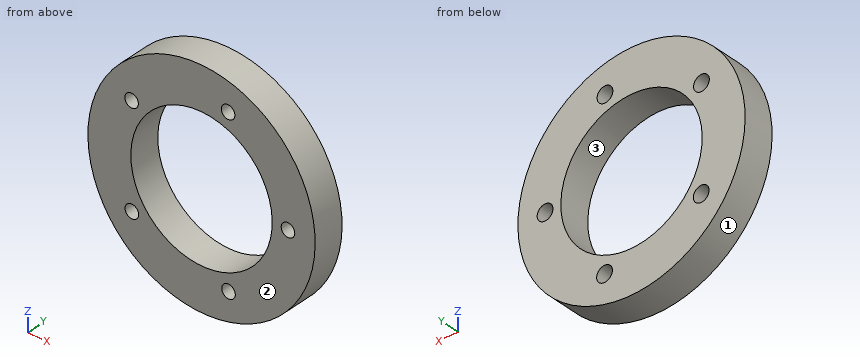
```python
from build123d import *

# Parameters (mm, degrees)
SKETCH1_R                    = 16.2
SKETCH1_R_2                  = 11.2
BOSS_EXTRUDE2_DEPTH          = 5
SKETCH2_R                    = 1.25
CUT_EXTRUDE1_DEPTH           = 5
CUT_EXTRUDE1_DRAFT           = -2
CUT_EXTRUDE1_PROFILE_2_DEPTH = 5
CUT_EXTRUDE1_PROFILE_2_DRAFT = -2
CUT_EXTRUDE1_PROFILE_3_DEPTH = 5
CUT_EXTRUDE1_PROFILE_3_DRAFT = -2
CUT_EXTRUDE1_PROFILE_4_DEPTH = 5
CUT_EXTRUDE1_PROFILE_4_DRAFT = -2
CUT_EXTRUDE1_PROFILE_5_DEPTH = 5
CUT_EXTRUDE1_PROFILE_5_DRAFT = -2
SKETCH3_R                    = 18
SKETCH3_R_2                  = 16
BOSS_EXTRUDE4_DEPTH          = 5


with BuildPart() as part:
    # Sketch1 → Boss-Extrude2 (new body)
    with BuildSketch(Plane(origin=(0, 0, 0), x_dir=(1, 0, 0), z_dir=(0, 1, 0))):
        with Locations(Location((0, 0, 0), (0, 0, 270))):
            Circle(SKETCH1_R)
        with Locations(Location((0, 0, 0), (0, 0, 270))):
            Circle(SKETCH1_R_2, mode=Mode.SUBTRACT)
    extrude(amount=BOSS_EXTRUDE2_DEPTH)


with BuildPart() as cut_extrude1_tool:
    # Sketch2 → Cut-Extrude1 (with draft: the straight prism first)
    with BuildSketch(Plane(origin=(0, 5, 0), x_dir=(1, 0, 0), z_dir=(0, 1, 0))):
        with Locations((-11.039322132, 8.113160104)):
            Circle(SKETCH2_R)
    extrude(amount=-CUT_EXTRUDE1_DEPTH)
    # Cut-Extrude1: the draft: its side faces are tilted about the plane it starts from
    cut_extrude1_sides = [cut_extrude1_tool.faces().sort_by_distance(p)[0] for p in [
        (-12.289322132, 2.5, -8.113160104),
    ]]
    draft(cut_extrude1_sides, Plane(origin=(0, 5, 0), x_dir=(1, 0, 0), z_dir=(0, 1, 0)), CUT_EXTRUDE1_DRAFT)


with BuildPart() as part_1:
    add(part.part)

    # Cut-Extrude1: cut by cut_extrude1_tool
    add(cut_extrude1_tool.part, mode=Mode.SUBTRACT)


with BuildPart() as cut_extrude1_profile_2_tool:
    # Sketch2 → Cut-Extrude1 profile 2 (with draft: the straight prism first)
    with BuildSketch(Plane(origin=(0, 5, 0), x_dir=(1, 0, 0), z_dir=(0, 1, 0))):
        with Locations((-11.083327892, -7.977724299)):
            Circle(SKETCH2_R)
    extrude(amount=-CUT_EXTRUDE1_PROFILE_2_DEPTH)
    # Cut-Extrude1 profile 2: the draft: its side faces are tilted about the plane it starts from
    cut_extrude1_profile_2_sides = [cut_extrude1_profile_2_tool.faces().sort_by_distance(p)[0] for p in [
        (-12.333327892, 2.5, 7.977724299),
    ]]
    draft(cut_extrude1_profile_2_sides, Plane(origin=(0, 5, 0), x_dir=(1, 0, 0), z_dir=(0, 1, 0)), CUT_EXTRUDE1_PROFILE_2_DRAFT)


with BuildPart() as part_2:
    add(part_1.part)

    # Cut-Extrude1 profile 2: cut by cut_extrude1_profile_2_tool
    add(cut_extrude1_profile_2_tool.part, mode=Mode.SUBTRACT)


with BuildPart() as cut_extrude1_profile_3_tool:
    # Sketch2 → Cut-Extrude1 profile 3 (with draft: the straight prism first)
    with BuildSketch(Plane(origin=(0, 5, 0), x_dir=(1, 0, 0), z_dir=(0, 1, 0))):
        with Locations((4.206414044, -12.991932999)):
            Circle(SKETCH2_R)
    extrude(amount=-CUT_EXTRUDE1_PROFILE_3_DEPTH)
    # Cut-Extrude1 profile 3: the draft: its side faces are tilted about the plane it starts from
    cut_extrude1_profile_3_sides = [cut_extrude1_profile_3_tool.faces().sort_by_distance(p)[0] for p in [
        (2.956414044, 2.5, 12.991932999),
    ]]
    draft(cut_extrude1_profile_3_sides, Plane(origin=(0, 5, 0), x_dir=(1, 0, 0), z_dir=(0, 1, 0)), CUT_EXTRUDE1_PROFILE_3_DRAFT)


with BuildPart() as part_3:
    add(part_2.part)

    # Cut-Extrude1 profile 3: cut by cut_extrude1_profile_3_tool
    add(cut_extrude1_profile_3_tool.part, mode=Mode.SUBTRACT)


with BuildPart() as cut_extrude1_profile_4_tool:
    # Sketch2 → Cut-Extrude1 profile 4 (with draft: the straight prism first)
    with BuildSketch(Plane(origin=(0, 5, 0), x_dir=(1, 0, 0), z_dir=(0, 1, 0))):
        with Locations((13.7, 0)):
            Circle(SKETCH2_R)
    extrude(amount=-CUT_EXTRUDE1_PROFILE_4_DEPTH)
    # Cut-Extrude1 profile 4: the draft: its side faces are tilted about the plane it starts from
    cut_extrude1_profile_4_sides = [cut_extrude1_profile_4_tool.faces().sort_by_distance(p)[0] for p in [
        (12.45, 2.5, 0),
    ]]
    draft(cut_extrude1_profile_4_sides, Plane(origin=(0, 5, 0), x_dir=(1, 0, 0), z_dir=(0, 1, 0)), CUT_EXTRUDE1_PROFILE_4_DRAFT)


with BuildPart() as part_4:
    add(part_3.part)

    # Cut-Extrude1 profile 4: cut by cut_extrude1_profile_4_tool
    add(cut_extrude1_profile_4_tool.part, mode=Mode.SUBTRACT)


with BuildPart() as cut_extrude1_profile_5_tool:
    # Sketch2 → Cut-Extrude1 profile 5 (with draft: the straight prism first)
    with BuildSketch(Plane(origin=(0, 5, 0), x_dir=(1, 0, 0), z_dir=(0, 1, 0))):
        with Locations((4.27761686, 13.043664873)):
            Circle(SKETCH2_R)
    extrude(amount=-CUT_EXTRUDE1_PROFILE_5_DEPTH)
    # Cut-Extrude1 profile 5: the draft: its side faces are tilted about the plane it starts from
    cut_extrude1_profile_5_sides = [cut_extrude1_profile_5_tool.faces().sort_by_distance(p)[0] for p in [
        (3.02761686, 2.5, -13.043664873),
    ]]
    draft(cut_extrude1_profile_5_sides, Plane(origin=(0, 5, 0), x_dir=(1, 0, 0), z_dir=(0, 1, 0)), CUT_EXTRUDE1_PROFILE_5_DRAFT)


with BuildPart() as part_5:
    add(part_4.part)

    # Cut-Extrude1 profile 5: cut by cut_extrude1_profile_5_tool
    add(cut_extrude1_profile_5_tool.part, mode=Mode.SUBTRACT)

    # Sketch3 → Boss-Extrude4 (add)
    with BuildSketch(Plane(origin=(0, 5, 0), x_dir=(1, 0, 0), z_dir=(0, 1, 0))):
        with Locations(Location((0, 0, 0), (0, 0, 270))):
            Circle(SKETCH3_R)
        Circle(SKETCH3_R_2, mode=Mode.SUBTRACT)
    extrude(amount=-BOSS_EXTRUDE4_DEPTH)


solid = part_5.part
```
The listing builds one solid part. Answer for the finished solid, in the listing's coordinates (mm). Face numbers are marked on the shaded views. Give positions to 0.01 mm unless a question says otherwise; leave off trailing zeros. Order: outer loops, then holes, each group sorted by start corner. A loop starts at its lowest first (then second) coordinate and runs counter-clockwise, first axis right, second up. Notation, with made-up numbers: M 62.25,70.25 L 94.25,70.25 A7 cw 94.25,74.25 Z; hole C 86.25,38.25 d9. An arc over 180 degrees is marked long. Put each result on its own line as item: value. Start each with the question number.
Item 1: Flat-ended cylindrical pins translate along their axes: P1, Ø2, axis at y = 2, z = -10.5, coming from the -X side; P2, Ø2, axis at x = -1.5, y = 4.5, coming from the -Z side; P3, Ø1.5, axis at x = 14, y = 4, coming from the +Z side. Find the tip coordinate at first contact, or state that the pin passes through.
Item 2: The part is cut by section A-A, the plane x = 0. Determine the outline of the cut face in (y, z), and give its area (3 significant figures).
Item 3: The part is cut by section D-D, the plane z = -4. Determine the outline of the cut face in (x, y), and give its area (3 significant figures).
Item 4: The part is cut by section C-C, the plane y = 3.25. Determine the outline of the cut face in (x, z), and give its area (3 significant figures).
Item 5: The part is cut by section B-B, the plane z = 0. Determine the outline of the cut face in (x, y).
Item 6: Find the intervals of material crossed by line 1 along X through (y, z) = (3.05, 0); line 2 along X through (y, z) = (1.15, 0); line 3 along X through (y, z) = (2.25, -6), in increasing order.
Item 7: For a pull along X with two mould halves and no side action, classify the marked faces 1, 2 and 3 as +X half, -X half, draft (parallel to the pull), parting line (faces both ways), or undercut.
Answer key:
1. P1: stops at x = -15.29
1. P2: stops at z = -17.99
1. P3: stops at z = 12.18
2. outline: M 0,-18 L 5,-18 L 5,-11.2 L 0,-11.2 Z; M 0,11.2 L 5,11.2 L 5,18 L 0,18 Z
2. area: 68.0 mm²
3. outline: M -17.55,0 L -10.46,0 L -10.46,5 L -17.55,5 Z; M 10.46,0 L 17.55,0 L 17.55,5 L 10.46,5 Z
3. area: 70.9 mm²
4. outline: C 0,0 d36; hole C -11.08,7.98 d2.38; hole C -11.04,-8.11 d2.38; hole C 0,0 d22.4; hole C 4.21,12.99 d2.38; hole C 4.28,-13.04 d2.38; hole C 13.7,0 d2.38
4. area: 602 mm²
5. outline: M -18,0 L -11.2,0 L -11.2,5 L -18,5 Z; M 11.2,0 L 12.62,0 L 12.45,5 L 11.2,5 Z; M 14.78,0 L 18,0 L 18,5 L 14.95,5 Z
6. line 1: x = -18 to -11.2, 11.2 to 12.52, 14.88 to 18
6. line 2: x = -18 to -11.2, 11.2 to 12.58, 14.82 to 18
6. line 3: x = -16.97 to -9.46, 9.46 to 16.97
7. face 1: parting line
7. face 2: draft
7. face 3: undercut
